from build123d import *

# Parameters (mm, degrees)
F0_R     = 1.75
F0_R_2   = 2
F1_DEPTH = 15


with BuildPart() as f1:
    # F0 (on Top) → F1 (new body)
    with BuildSketch(Plane.XY):
        with BuildLine():
            ThreePointArc((4.4705081946, 34.1311327705), (3.5950567719, 34.6111450962), (2.6105643925, 34.7772829339))
            Line((2.6105643925, 34.7772829339), (-45.2081770897, 34.7772829339))
            ThreePointArc((-45.2081770897, 34.7772829339), (-47.3294974333, 33.8986032775), (-48.2081770897, 31.7772829339))
            Line((-48.2081770897, 31.7772829339), (-48.2081770897, 29.7772829339))
            ThreePointArc((-48.2081770897, 29.7772829339), (-47.3294974333, 27.6559625904), (-45.2081770897, 26.7772829339))
            Line((-45.2081770897, 26.7772829339), (-21.2081770897, 26.7772829339))
            ThreePointArc((-21.2081770897, 26.7772829339), (-19.0868567461, 25.8986032775), (-18.2081770897, 23.7772829339))
            Line((-18.2081770897, 23.7772829339), (-18.2081770897, -24.2227170661))
            ThreePointArc((-18.2081770897, -24.2227170661), (-19.0868567461, -26.3440374096), (-21.2081770897, -27.2227170661))
            Line((-21.2081770897, -27.2227170661), (-45.2081770897, -27.2227170661))
            ThreePointArc((-45.2081770897, -27.2227170661), (-47.3294974333, -28.1013967225), (-48.2081770897, -30.2227170661))
            Line((-48.2081770897, -30.2227170661), (-48.2081770897, -32.2227170661))
            ThreePointArc((-48.2081770897, -32.2227170661), (-47.3294974333, -34.3440374096), (-45.2081770897, -35.2227170661))
            Line((-45.2081770897, -35.2227170661), (28.7918229103, -35.2227170661))
            ThreePointArc((28.7918229103, -35.2227170661), (30.9131432539, -34.3440374096), (31.7918229103, -32.2227170661))
            Line((31.7918229103, -32.2227170661), (31.7918229103, 11.0896125673))
            ThreePointArc((31.7918229103, 11.0896125673), (31.4918072997, 12.3973144816), (30.6517667124, 13.4434624038))
            Line((30.6517667124, 13.4434624038), (13.7918229103, 26.7657005056))
            Line((13.7918229103, 26.7657005056), (13.7771647808, 26.7772829339))
            Line((13.7771647808, 26.7772829339), (4.4705081946, 34.1311327705))
        make_face()
        with Locations((-44.7081770897, -31.2227170661)):
            Circle(F0_R, mode=Mode.SUBTRACT)
        with Locations((-22.7081770897, -31.2227170661)):
            Circle(F0_R, mode=Mode.SUBTRACT)
        with Locations((21.7918229103, -30.2227170661)):
            Circle(F0_R_2, mode=Mode.SUBTRACT)
        with BuildLine():
            Line((10.7918229103, -27.2227170661), (-7.2081770897, -27.2227170661))
            ThreePointArc((-7.2081770897, -27.2227170661), (-9.3294974333, -26.3440374096), (-10.2081770897, -24.2227170661))
            Line((-10.2081770897, -24.2227170661), (-10.2081770897, -5.0720059582))
            ThreePointArc((-10.2081770897, -5.0720059582), (-8.5158790041, -2.3720215688), (-5.3482332876, -2.7181561216))
            Line((-5.3482332876, -2.7181561216), (12.6517667124, -16.941233532))
            ThreePointArc((12.6517667124, -16.941233532), (13.4918072997, -17.9873814542), (13.7918229103, -19.2950833685))
            Line((13.7918229103, -19.2950833685), (13.7918229103, -24.2227170661))
            ThreePointArc((13.7918229103, -24.2227170661), (12.9131432539, -26.3440374096), (10.7918229103, -27.2227170661))
        make_face(mode=Mode.SUBTRACT)
        with BuildLine():
            ThreePointArc((18.8984889537, -6.2227170661), (19.7771686101, -4.1013967225), (21.8984889537, -3.2227170661))
            Line((21.8984889537, -3.2227170661), (23.8984889537, -3.2227170661))
            ThreePointArc((23.8984889537, -3.2227170661), (26.0198092973, -4.1013967225), (26.8984889537, -6.2227170661))
            Line((26.8984889537, -6.2227170661), (26.8984889537, -20.2227170661))
            ThreePointArc((26.8984889537, -20.2227170661), (26.0198092973, -22.3440374096), (23.8984889537, -23.2227170661))
            Line((23.8984889537, -23.2227170661), (21.8984889537, -23.2227170661))
            ThreePointArc((21.8984889537, -23.2227170661), (19.7771686101, -22.3440374096), (18.8984889537, -20.2227170661))
            Line((18.8984889537, -20.2227170661), (18.8984889537, -6.2227170661))
        make_face(mode=Mode.SUBTRACT)
        with Locations((-44.7081770897, 30.8822728693)):
            Circle(F0_R, mode=Mode.SUBTRACT)
        with Locations((-22.7081770897, 30.7772829339)):
            Circle(F0_R, mode=Mode.SUBTRACT)
        with BuildLine():
            ThreePointArc((-10.2081770897, 23.7772829339), (-9.3294974333, 25.8986032775), (-7.2081770897, 26.7772829339))
            Line((-7.2081770897, 26.7772829339), (2.1063956214, 26.7772829339))
            ThreePointArc((2.1063956214, 26.7772829339), (3.4809139878, 26.4438723774), (4.5499130653, 25.5177491075))
            Line((4.5499130653, 25.5177491075), (13.2353403542, 13.3238935696))
            ThreePointArc((13.2353403542, 13.3238935696), (13.6493176462, 12.4970596164), (13.7918229103, 11.583427396))
            Line((13.7918229103, 11.583427396), (13.7918229103, -0.1256085036))
            ThreePointArc((13.7918229103, -0.1256085036), (12.0995248247, -2.825592893), (8.9318791082, -2.4794583402))
            Line((8.9318791082, -2.4794583402), (-9.0681208918, 11.7436190702))
            ThreePointArc((-9.0681208918, 11.7436190702), (-9.9081614791, 12.7897669924), (-10.2081770897, 14.0974689067))
            Line((-10.2081770897, 14.0974689067), (-10.2081770897, 23.7772829339))
        make_face(mode=Mode.SUBTRACT)
        with Locations((21.7918229103, 3.7772829339)):
            Circle(F0_R_2, mode=Mode.SUBTRACT)
    extrude(amount=F1_DEPTH)


solid = f1.part
Work out the finished part from the listing and answer in its coordinate system (mm). A direction names the side the tool comes from. Give positions to 0.01 mm unless a question says otherwise; leave off trailing zeros. Loops run counter-clockwise (first coordinate to the right, second up) from the corner with the lowest first, then second, coordinate; pieces in that order, holes last. Notation, with made-up numbers: (34.5, 49) - (53.5, 49) arc R22 cw to (53.5, 85) - close; hole circle Ø4 at (-8.5, 63). An arc over 180 degrees is marked (long way). Answer in a Markdown table with one row per item. Add a question column.
Q1. Consider line 1 along Y through (x, z) = (-36.5, 3.75); line 2 along Y through (x, z) = (-21.5, 14.25); line 3 along X through (y, z) = (-15.5, 12.75). Determine where each line is inside the solid, lowest interval first.
Q2. Determine the mould class of faces 4 (the flat face through (23, -23.223, 7)), 5 (the cylindrical face through (3.608, 34.607, 7.395)), 6 (the flat face through (0, 0, 0)) for opening direction Y: released by +Y, released by -Y, zero draft, split by the parting line, or undercut.
Q3. The part is cut by section C-C (x = -3). Determine the outline of the cut face in (y, z).
Q4. A tool of negligible diameter and unlimited length cuts with its end or side. For faces 1 (the flat face through (-18.208, 0, 7)), 2 (the flat face through (-48.208, 31, 7)), 3 (the cylindrical face through (26, -4.08, 7.4)), from which of +Z, -Z, +X, -X, +Y, -Y can it reach the whole face along a straight path? Write none if from no direction.
Q5. Each of these flat-tipped pins is pushed along its axis until it touches: P1, Ø1.6, axis at x = 23, z = 6, coming from the +Y side; P2, Ø3, axis at x = -22.71, y = -31.22, coming from the -Z side; P3, Ø5, axis at y = -11, z = 6, coming from the -X side; P4, Ø5, axis at y = 26.5, z = 9.5, coming from the -X side. Where does it stop, or does it pass through?
Q6. The part is cut by section B-B (y = 17). Determine the outline of the cut face in (x, z).
Q7. The part is cut by section D-D (y = -7.5). Determine the outline of the cut face in (x, z).
Q8. The part is cut by section A-A (x = -42). Determine the outline of the cut face in (y, z).
Solution:
| question | item | result |
|---|---|---|
| 1 | line 1 | y = -35.22 to -27.22, 26.78 to 34.78 |
| 1 | line 2 | y = -35.22 to -32.49, -29.96 to -27.22, 26.78 to 29.51, 32.04 to 34.78 |
| 1 | line 3 | x = -18.21 to -10.21, 10.83 to 18.9, 26.9 to 31.79 |
| 2 | face 4 | undercut |
| 2 | face 5 | released by +Y |
| 2 | face 6 | zero draft |
| 3 | outline | (-35.22, 0) - (-27.22, 0) - (-27.22, 15) - (-35.22, 15) - close; (-4.57, 0) - (6.95, 0) - (6.95, 15) - (-4.57, 15) - close; (26.78, 0) - (34.78, 0) - (34.78, 15) - (26.78, 15) - close |
| 4 | face 1 | +Z, -Z, -X |
| 4 | face 2 | +Z, -Z, -X, +Y, -Y |
| 4 | face 3 | +Z, -Z |
| 5 | P1 | stops at y = 20.12 |
| 5 | P2 | passes through |
| 5 | P3 | stops at x = -18.21 |
| 5 | P4 | stops at x = -48.11 |
| 6 | outline | (-18.21, 0) - (-10.21, 0) - (-10.21, 15) - (-18.21, 15) - close; (10.62, 0) - (26.15, 0) - (26.15, 15) - (10.62, 15) - close |
| 7 | outline | (-18.21, 0) - (-10.21, 0) - (-10.21, 15) - (-18.21, 15) - close; (0.7, 0) - (18.9, 0) - (18.9, 15) - (0.7, 15) - close; (26.9, 0) - (31.79, 0) - (31.79, 15) - (26.9, 15) - close |
| 8 | outline | (-35.22, 0) - (-27.22, 0) - (-27.22, 15) - (-35.22, 15) - close; (26.78, 0) - (34.78, 0) - (34.78, 15) - (26.78, 15) - close |
